Part model, mm, in its own coordinate system. A direction names the side the tool comes from. Round coordinates to 2 decimals unless told otherwise and drop trailing zeros. Answer as a JSON object with one key per item and string values. Group by question number.
1. Which spindle directions (+Z, -Z, +X, -X, +Y, -Y) get a long thin tool onto all of the face, cutting with end or side? Do faces 1 (the face through (-231.445, 215.979, 8.381)), 2 (the face through (190.651, -185.043, 12.93)). Say none if no direction does.
2. Two-plate mould, pull along X, no slides. Class faces 3 (the face through (-231.445, -215.979, 8.619)), 4 (the face through (240, 3, 8)), 5 (the face through (-3, 225, 8)), 6 (the face through (-189.17, 190.26, 5.52)): +X half, -X half, draft (parallel to the pull), parting line (faces both ways), or undercut.
3. Drill centre lines: line 1 (Y direction, x = 190, z = 11.5); line 2 (X direction, y = 190, z = 15); line 3 (X direction, y = 187, z = 14.25). Where is each one in solid material? Low to high. Write a range as from..to.
from build123d import *

# Parameters (mm, degrees)
P_IDAT_VYSUNUT_M1_DEPTH      = 18
D_RY_PRO_KOL_K_10_0MM1_D     = 10
D_RY_PRO_KOL_K_10_0MM1_DEPTH = 10
D_RY_PRO_KOL_K_10_0MM1_TIP   = 3.004303095
ZAOBLIT1_R                   = 30
ZAOBLIT2_R                   = 1


with BuildPart() as part:
    # Skica1 → Přidat vysunutím1 (new body)
    with BuildSketch(Plane.XY):
        with BuildLine():
            Line((-210, 225), (210, 225))
            ThreePointArc((210, 225), (231.213203436, 216.213203436), (240, 195))
            Line((240, 195), (240, -195))
            ThreePointArc((240, -195), (231.213203436, -216.213203436), (210, -225))
            Line((210, -225), (-240, -225))
            Line((-240, -225), (-240, 195))
            ThreePointArc((-240, 195), (-231.213203436, 216.213203436), (-210, 225))
        make_face()
    extrude(amount=P_IDAT_VYSUNUT_M1_DEPTH)

    # Díry pro kolík, Ø10.0mm1
    with Locations(Plane.XY.offset(18)):
        with Locations((-190, 190), (190, 190), (190, -190), (-190, -190)):
            Hole(D_RY_PRO_KOL_K_10_0MM1_D / 2, depth=D_RY_PRO_KOL_K_10_0MM1_DEPTH)
            with Locations((0, 0, -(D_RY_PRO_KOL_K_10_0MM1_DEPTH + D_RY_PRO_KOL_K_10_0MM1_TIP / 2))):  # 118° drill point
                Cone(0, D_RY_PRO_KOL_K_10_0MM1_D / 2, D_RY_PRO_KOL_K_10_0MM1_TIP, mode=Mode.SUBTRACT)

    # Zaoblit1
    zaoblit1_edges = [part.edges().sort_by_distance(p)[0] for p in [
        (-240, -225, 9),
    ]]
    fillet(zaoblit1_edges, radius=ZAOBLIT1_R)

    # Zaoblit2
    zaoblit2_edges = [part.edges().sort_by_distance(p)[0] for p in [
        (240, 0, 18),
        (231.213203436, 216.213203436, 18),
        (0, 225, 18),
        (-231.213203436, 216.213203436, 18),
        (-240, 0, 18),
        (0, -225, 18),
        (-231.213203436, -216.213203436, 18),
        (231.213203436, -216.213203436, 18),
    ]]
    fillet(zaoblit2_edges, radius=ZAOBLIT2_R)


solid = part.part
Worked answers:
{
 "1": {"face 1": "+Z, -Z, -X, +Y", "face 2": "+Z"},
 "2": {"face 3": "-X half", "face 4": "+X half", "face 5": "draft", "face 6": "undercut"},
 "3": {"line 1": "y = -225..-195, -185..185, 195..225", "line 2": "x = -240..-195, -185..185, 195..240", "line 3": "x = -240..-194, -186..186, 194..240"}
}
